Verification items for the finished model (mm, model axes). Face numbers are marked on the shaded views. Give positions to 0.01 mm unless a question says otherwise; leave off trailing zeros. Order: outer loops, then holes, each group sorted by start corner. A loop starts at its lowest first (then second) coordinate and runs counter-clockwise, first axis right, second up. Notation, with made-up numbers: (43.25, -22) -> (68.25, -22) arc R29 ccw to (68.25, 4) -> close; hole circle Ø11 at (50, 41). An arc over 180 degrees is marked (long way). Return JSON: item names as keys, results as strings. Group by question number.
(1) Thickness scan on line 1 along X through (y, z) = (-8.5, -1.25); line 2 along Z through (x, y) = (-38, -6.75); line 3 along X through (y, z) = (-10.25, -2.25). Record the ranges inside material, lowest first.
(2) Depth check by flat-ended pin: pin 1 Ø1 at (x, y) = (-27, -16) entering from -Z; pin 2 Ø1.5 at (y, z) = (-11, 0.5) entering from -X; pin 3 Ø8 at (x, y) = (-63, -5) entering from +Z. Enter the tip coordinate at first touch or a pass-through.
(3) Release check for a two-part mould opening along Z. For the marked faces 1, 2 and 3 record: pulls with the +Z half, pulls with the -Z half, needs draft (parallel to the pull), parting line crosses it, or undercut.
(4) Cross-section at A-A on z = -2. Enter the section's corners in (x, y), then the cut area to 3 significant figures.
(5) Cross-section at B-B on y = -9. Enter the section's corners in (x, z).
(6) Cross-section at D-D on z = 1.75. Enter the section's corners in (x, y), then the cut area to 3 significant figures.
(7) Cross-section at C-C on x = -36. Enter the section's corners in (y, z), then the cut area to 3 significant figures.
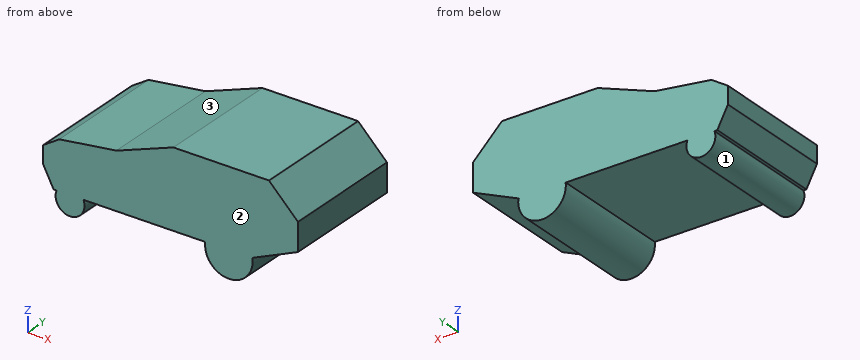
from build123d import *

# Parameters (mm, degrees)
F4_DEPTH = 26.0096


with BuildPart() as f4:
    # F3 (on Front) → F4 (new body)
    with BuildSketch(Plane.XZ):
        with BuildLine():
            Line((-15.027259, 4.264493), (-15.027259, 10.153553))
            Line((-15.027259, 10.153553), (-21.119392, 16.245686))
            Line((-21.119392, 16.245686), (-41.223429, 16.245686))
            Line((-41.223429, 16.245686), (-53.204622, 11.778122))
            Line((-53.204622, 11.778122), (-65.185815, 10.153553))
            Line((-65.185815, 10.153553), (-68.638019, 7.919772))
            Line((-68.638019, 7.919772), (-68.638019, 4.264493))
            Line((-68.638019, 4.264493), (-66.404238, 0))
            Line((-66.404238, 0), (-65.795027, 0))
            ThreePointArc((-65.795027, 0), (-62.952032, -4.125348), (-60.109038, 0))
            Line((-60.109038, 0), (-34.520175, 0))
            ThreePointArc((-34.520175, 0), (-29.543368, -5.586779), (-24.566561, 0))
            Line((-24.566561, 0), (-24.774671, 0))
            Line((-24.774671, 0), (-15.027259, 4.264493))
        make_face()
    extrude(amount=F4_DEPTH)


solid = f4.part
Verdict:
{
 "1": {"line 1": "-65.99 to -59.91, -34.51 to -24.58", "line 2": "0 to 16.25", "line 3": "-65.76 to -60.14, -34.27 to -24.82"},
 "2": {"pin 1": "z = -5.15", "pin 2": "x = -67.06", "pin 3": "z = 10.99"},
 "3": {"face 1": "undercut", "face 2": "needs draft", "face 3": "pulls with the +Z half"},
 "4": {"outline": "(-65.85, -26.01) -> (-60.05, -26.01) -> (-60.05, 0) -> (-65.85, 0) -> close; (-34.35, -26.01) -> (-24.74, -26.01) -> (-24.74, 0) -> (-34.35, 0) -> close", "area": "401 mm²"},
 "5": {"outline": "(-68.64, 4.26) -> (-66.4, 0) -> (-65.8, 0) arc R3.04 ccw (long way) to (-60.11, 0) -> (-34.52, 0) arc R5.01 ccw (long way) to (-24.57, 0) -> (-24.77, 0) -> (-15.03, 4.26) -> (-15.03, 10.15) -> (-21.12, 16.25) -> (-41.22, 16.25) -> (-53.2, 11.78) -> (-65.19, 10.15) -> (-68.64, 7.92) -> close"},
 "6": {"outline": "(-67.32, -26.01) -> (-20.77, -26.01) -> (-20.77, 0) -> (-67.32, 0) -> close", "area": "1,210 mm²"},
 "7": {"outline": "(-26.01, 0) -> (0, 0) -> (0, 16.25) -> (-26.01, 16.25) -> close", "area": "423 mm²"}
}
